Autodesk Inventor part; units mm, degrees
ref_plane "Work Plane2" through (-37, -13, 19) normal (0, 0, -1) x (0, 1, 0)
ref_plane "YZ Plane" through (0, 0, 0) normal (1, 0, 0) x (0, 1, 0)
ref_plane "XZ Plane" through (0, 0, 0) normal (0, 1, 0) x (-1, 0, 0)
ref_plane "Work Plane1" through (0, 0, 0) normal (0, 0, 1) x (1, 0, 0)
ref_plane "Work Plane2" through (-37, -13, 19) normal (0, 0, -1) x (0, 1, 0)
sketch "Sketch1" plane through (0, 0, 0) normal (0, 0, 1) x (1, 0, 0)
  line L0 (35, 13) -> (35, -13)
  line L1 (20, 0) -> (20, 13)
  circle A0 centre (27.5, 9) radius 2
  circle A1 centre (27.5, -9) radius 2
  line L2 (35, 13) -> (20, 13)
  line L3 (35, -13) -> (24.5, -13)
  line L4 (24.5, -13) -> (24.5, -6)
  line L5 (20, 0) -> (20, 13)
  line L6 (-60.2, 0) -> (60.2, 0) construction
  line L7 (35, 13.1624) -> (35, -13.1624) construction
  circle A2 centre (24.5, 0) radius 2.5
  line L8 (20, -13.1624) -> (20, 13.1624) construction
  line L9 (24.5, -6) -> (20, 0)
  point P0 (0, 0)
  dimension "d1" = 3
  dimension "d26" = 26
  dimension "d29" = 7
extrude "Extrusion1" add sketch "Sketch1" along normal up to surface (19 mm away)
ref_plane "Work Plane4" through (-0.8627, 0, 12) normal (0, 0, 1) x (1, 0, 0)
sketch "Sketch4" plane through (-0.8627, 0, 12) normal (0, 0, 1) x (1, 0, 0)
  circle A0 centre (28.3627, 9) radius 2 construction
  circle A1 centre (25.3627, 0) radius 2.5 construction
  circle A2 centre (28.3627, -9) radius 2 construction
  circle A3 centre (28.3627, -9) radius 2 construction
  circle A4 centre (28.3627, 9) radius 2 construction
  line L0 (35.8627, -13) -> (35.8627, 13) construction
  line L1 (35.8627, 13) -> (20.8627, 13) construction
  line L2 (20.8627, 13) -> (20.8627, 0) construction
  line L3 (25.3627, -6) -> (25.3627, -13) construction
  line L4 (25.3627, -13) -> (35.8627, -13) construction
  line L5 (20.8627, 8.7113) -> (35.8627, 0.0511) construction
  line L6 (35.8627, -13) -> (35.8627, 13) construction
  line L7 (-2.1421, -20.2045) -> (16.8579, 12.7045) construction
  line L8 (35.8627, 0.0511) -> (20.8627, 8.7113)
  line L9 (20.8627, 0) -> (25.3627, -6)
  point P0 (0.8627, 0)
  dimension "d6" = 4
ref_plane "Work Plane8" through (43.6603, -4.9489, 12) normal (0.866, -0.5, 0) x (0.5, 0.866, 0)
ref_plane "Work Plane7" through (35, 0.0511, 12) normal (0.866, -0.5, 0) x (0.5, 0.866, 0)
sketch "Sketch7" plane through (43.6603, -4.9489, 12) normal (0.866, -0.5, 0) x (0.5, 0.866, 0)
  point P0 (-17.5442, -12)
  point P1 (0, 0)
hole "Hole2" at (43.6603, -4.9489, 12) direction (-0.866, 0.5, 0) diameter 2.459 end through all
fillet "Fillet1" radius 2 4 edges at (35, 13, 9.5) (20, 13, 9.5) (24.5, -13, 9.5) (35, -13, 9.5)
Source: CAD feature listing. Evaluate the final solid. Frame: model axes, mm. A direction names the side the tool comes from. Round coordinates to 2 decimals unless told otherwise and drop trailing zeros. Loops run counter-clockwise (first coordinate to the right, second up) from the corner with the lowest first, then second, coordinate; pieces in that order, holes last. Notation, with made-up numbers: (-15, 15.5) - (-4, 15.5) arc R23 cw to (-4, 31.5) - close; hole circle Ø3 at (31, 24.5). An arc over 180 degrees is marked (long way). Write item = value, one per line. Start each with the question number.
(1) Section query A-A, the plane z = 3. Output: boundary loops of the cut face in (x, y).
(2) Ray query, line 1 along Y through (x, z) = (27.5, 5.5); line 2 along Y through (x, z) = (26, 7.5); line 3 along Y through (x, z) = (26.25, 7). Return the intervals inside material, ascending. Write a range as from..to.
(3) Set-up query: faces 1 (the face through (24.5, -9, 9)), 2 (the face through (22, 0, 9)). Return all of +Z, -Z, +X, -X, +Y, -Y with unobstructed straight access to the full face (end or side cutting, diameter ignored); none if empty.
(4) Section query B-B, the plane x = 27.5. State how many separate pieces and enclosed holes the cut face has, plus the area to 3 significant figures.
(5) Pull-direction query (Z, two-part tool) for faces 3 (the face through (22.28, -3.04, 9.37)), 4 (the face through (29, 0, 0)), 5 (the face through (27.76, 5.09, 12.98)); classes: +Z half, -Z half, draft (parallel to the pull), parting line (faces both ways), or undercut.
(6) Pin query (flat end, axial travel): pin 1 (5.5 mm diameter, centred on y = -8.5, z = 9.5, fed in from -X). Return the tip coordinate at first contact, or that it passes through.
Conclusion:
q1.outline = (20, 0) - (24.5, -6) - (24.5, -11) arc R2 ccw to (26.5, -13) - (33, -13) arc R2 ccw to (35, -11) - (35, 11) arc R2 ccw to (33, 13) - (22, 13) arc R2 ccw to (20, 11) - close; hole circle Ø5 at (24.5, 0); hole circle Ø4 at (27.5, -9); hole circle Ø4 at (27.5, 9)
q2.line_1 = -13..-11, -7..7, 11..13
q2.line_2 = -12.94..-10.32, -7.68..-2, 2..7.68, 10.32..13
q2.line_3 = -12.98..-10.56, -7.44..-1.79, 1.79..7.44, 10.56..13
q3.face_1 = +Z, -Z, -X, -Y
q3.face_2 = +Z, -Z
q4.separate_pieces = 3
q4.enclosed_holes = 1
q4.area = 337 mm2
q5.face_3 = draft
q5.face_4 = -Z half
q5.face_5 = undercut
q6.pin_1 = 24.31
